For this review, use the dimensioned drawing (mm, ordinates from the lowest corner) and the shaded views. A direction names the side the tool comes from. Give positions to 0.01 mm unless a question says otherwise; leave off trailing zeros. Write each loop counter-clockwise with the first axis right and the second up, starting at its lowest first coordinate (ties: lowest second). Pieces come first, ordered by that corner, then holes. Notation, with made-up numbers: M 50.25,-19.75 L 57.25,-19.75 A11 ccw 57.25,1.25 Z; hole C 51,-27 d2. An arc over 180 degrees is marked long. Answer in a Markdown table with one row per item.
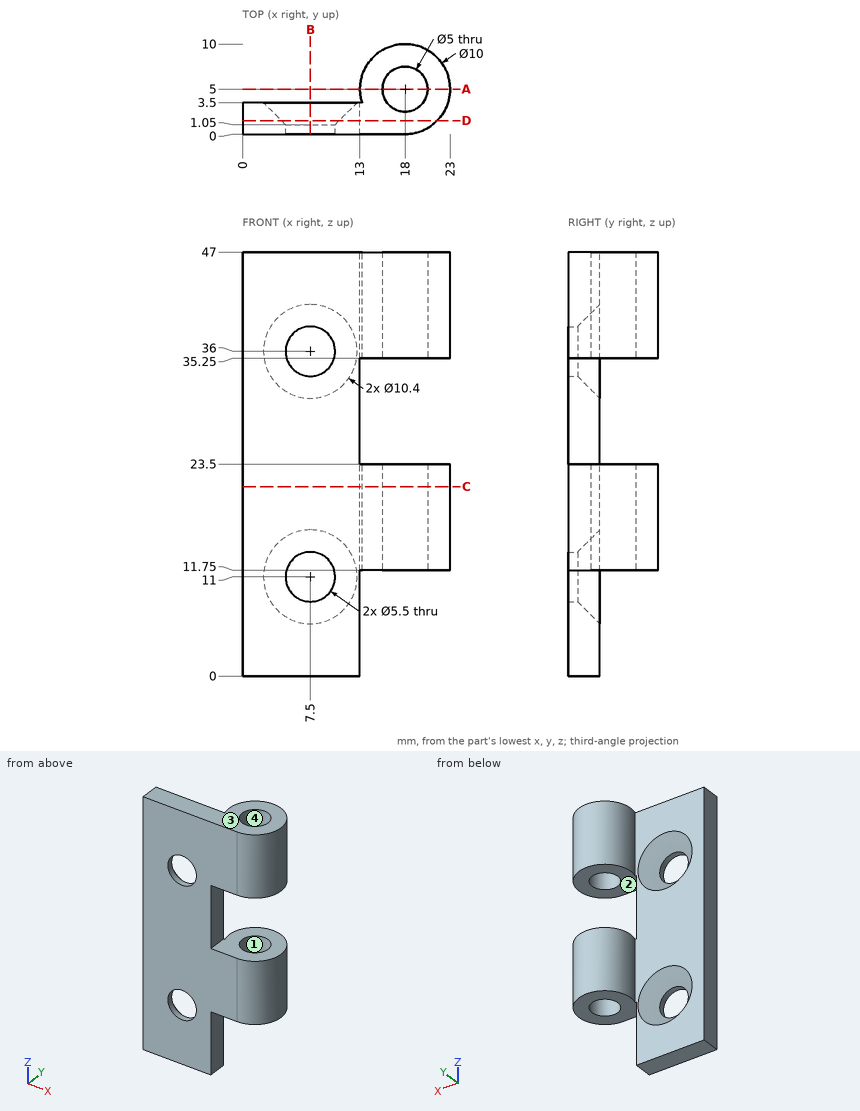
1) Add section A-A (y = 5). Write out the cut boundary in (x, z), and give its area (4 significant figures).
Geometry says:
| item | result |
|---|---|
| outline | M 13,11.75 L 15.5,11.75 L 15.5,23.5 L 13,23.5 Z; M 13,35.25 L 15.5,35.25 L 15.5,47 L 13,47 Z; M 20.5,11.75 L 23,11.75 L 23,23.5 L 20.5,23.5 Z; M 20.5,35.25 L 23,35.25 L 23,47 L 20.5,47 Z |
| area | 117.5 mm^2 |
2) Add section D-D (y = 1.5). Write out the cut boundary in (x, z).
Geometry says:
| item | result |
|---|---|
| outline | M 0,0 L 13,0 L 13,11.75 L 21.57,11.75 L 21.57,23.5 L 13,23.5 L 13,35.25 L 21.57,35.25 L 21.57,47 L 0,47 Z; hole C 7.5,11 d6.4; hole C 7.5,36 d6.4 |
3) The part is to be moulded in two halves that separate along X. For the marked faces 3 and 4, say which applies: released by +X, released by -X, zero draft, split by the parting line, or undercut.
Geometry says:
| item | result |
|---|---|
| face 3 | zero draft |
| face 4 | undercut |
4) Add section B-B (x = 7.5). Write out the cut boundary in (y, z).
Geometry says:
| item | result |
|---|---|
| outline | M 0,0 L 3.5,0 L 3.5,5.8 L 1.05,8.25 L 0,8.25 Z; M 0,13.75 L 1.05,13.75 L 3.5,16.2 L 3.5,30.8 L 1.05,33.25 L 0,33.25 Z; M 0,38.75 L 1.05,38.75 L 3.5,41.2 L 3.5,47 L 0,47 Z |
5) Add section C-C (z = 21). Write out the cut boundary in (x, y), and give its area (3 significant figures).
Geometry says:
| item | result |
|---|---|
| outline | M 0,0 L 18,0 A5 ccw long 13.23,3.5 L 0,3.5 Z; hole C 18,5 d5 |
| area | 110 mm^2 |
6) To check wall thickness, follow probe 1 along Z at (x, y) = (7.5, 0.7); probe 2 along Z at (x, y) = (13.75, 4.75); probe 3 along Y at (x, z) = (18, 17.5). State the ranges of each line that lie inside material, in increasing order. Write a range as [from, to].
Geometry says:
| item | result |
|---|---|
| probe 1 | [0, 8.25], [13.75, 33.25], [38.75, 47] |
| probe 2 | [11.75, 23.5], [35.25, 47] |
| probe 3 | [0, 2.5], [7.5, 10] |
7) For the marked faces 1 and 2, list the 3-axis set-ups (+Z, -Z, +X, -X, +Y, -Y) from which the entire face can be reached by the end or side of a thin tool; tool diameter is ignored.
Geometry says:
| item | result |
|---|---|
| face 1 | +Z, -Z |
| face 2 | +X, +Y, -Y |
8) Insertion check: P1, Ø4.5, axis at x = 7.5, z = 11, coming from the -Y side; P2, Ø8, axis at x = 5.5, z = 42, coming from the +Y side; P3, Ø4, axis at y = 7, z = 23.5, coming from the -X side; P4, Ø4, axis at y = 1.5, z = 31.5, coming from the +X side. Each pin has a flat end and moves straight along its axis. Give the tip position at first contact, or say it passes through.
Geometry says:
| item | result |
|---|---|
| P1 | through |
| P2 | y = 3.5 |
| P3 | x = 13 |
| P4 | x = 13 |
